Geometry: final body of the model. Coordinates: model frame, mm. A direction names the side the tool comes from. Give positions to 0.01 mm unless a question says otherwise; leave off trailing zeros. Order: outer loops, then holes, each group sorted by start corner. A loop starts at its lowest first (then second) coordinate and runs counter-clockwise, first axis right, second up. Notation, with made-up numbers: (27.5, 37.25) -> (55.5, 37.25) arc R28 cw to (55.5, 58.25) -> close; hole circle Ø11 at (81.25, -37.5). An arc over 180 degrees is marked (long way). One line per question, with ' | ' between items. Start each with the question number.
(1) Mould query, pull axis Y, two halves, no side actions, for faces 6 (the face through (18.71, 62, 25)), 7 (the face through (53, -14.773, 24)), 8 (the face through (53, 23.364, 17)), 9 (the face through (-11, 68.064, 17)). Classes: +Y half, -Y half, draft (parallel to the pull), parting line (faces both ways), or undercut.
(2) Section B-B (y = -19.5). Return loops of the section in (x, z).
(3) Section A-A (z = 5). Return loops of the section in (x, y), then the cut area to 3 significant figures.
(4) Ray query, L1, parallel to Y at x = -70, z = 18.5; L2, parallel to Y at x = -71, z = 3; L3, parallel to X at y = 50, z = 27. Return the intervals inside material, ascending.
(5) Set-up query: faces 1 (the face through (55, 33.196, 17)), 2 (the face through (-56.21, 50, 17)), 3 (the face through (-73, 23.228, 17)), 4 (the face through (-68.23, -26, 23)), 5 (the face through (-78.23, 26, 17)). Return all of +Z, -Z, +X, -X, +Y, -Y with unobstructed straight access to the full face (end or side cutting, diameter ignored); none if empty.
(6) Section C-C (x = -40.5). Return loops of the section in (y, z).
(7) First-contact query: pin 1 Ø7.5 at (y, z) = (18.5, 17) entering from +X; pin 2 Ø1 at (y, z) = (-20, 27) entering from -X; pin 3 Ø3.5 at (y, z) = (30, 16) entering from -X; pin 4 Ø8.5 at (y, z) = (53, 22.5) entering from -X. Flat tips, straight axial feed; report the tip coordinate or a pass-through.
```python
from build123d import *

# Parameters (mm, degrees)
SKETCH_1_W           = 136.18
SKETCH_1_H           = 105.19
EXTRUDE_1_DEPTH      = 34
SKETCH_3_W           = 39.24
SKETCH_3_H           = 34
CUT_EXTRUDE_1_DEPTH  = 28.96
SKETCH_4_W           = 17.22
SKETCH_4_H           = 34
EXTRUDE_2_DEPTH      = 17.22
SKETCH_5_W           = 19.62
SKETCH_5_H           = 34
EXTRUDE_3_DEPTH      = 17.22
SKETCH_6_W           = 34
SKETCH_6_H           = 4.24
CUT_EXTRUDE_2_DEPTH  = 5
SKETCH_7_W           = 34
SKETCH_7_H           = 7
CUT_EXTRUDE_4_DEPTH  = 10
SKETCH_9_W           = 19.62
SKETCH_9_H           = 13.59
EXTRUDE_4_DEPTH      = 11
SKETCH_10_W          = 17.22
SKETCH_10_H          = 13.58
EXTRUDE_5_DEPTH      = 11
SKETCH_11_W          = 34
SKETCH_11_H          = 5
CUT_EXTRUDE_7_DEPTH  = 5
SKETCH_13_W          = 33.75
SKETCH_13_H          = 7
CUT_EXTRUDE_9_DEPTH  = 10
SKETCH_15_W          = 10
SKETCH_15_H          = 7
CUT_EXTRUDE_10_DEPTH = 10
SKETCH_16_W          = 21.544160933
SKETCH_16_H          = 22.857254915
CUT_EXTRUDE_11_DEPTH = 10
SKETCH_18_W          = 19.981240116
SKETCH_18_H          = 22.352912948
CUT_EXTRUDE_12_DEPTH = 10


with BuildPart() as part:
    # 草图1 → 凸台-拉伸1 (new body)
    with BuildSketch(Plane.XY):
        with Locations((-10.139734918, 15.469024107)):
            Rectangle(SKETCH_1_W, SKETCH_1_H)
    extrude(amount=EXTRUDE_1_DEPTH)

    # 草图3 → 切除-拉伸1 (cut)
    with BuildSketch(Plane(origin=(0, 68.064024107, 0), x_dir=(1, 0, 0), z_dir=(0, 1, 0))):
        with Locations((-58.609734918, -17)):
            Rectangle(SKETCH_3_W, SKETCH_3_H)
        with Locations((38.330265082, -17)):
            Rectangle(SKETCH_3_W, SKETCH_3_H)
    extrude(amount=-CUT_EXTRUDE_1_DEPTH, mode=Mode.SUBTRACT)

    # 草图4 → 凸台-拉伸2 (add)
    with BuildSketch(Plane(origin=(0, 39.104024107, 0), x_dir=(1, 0, 0), z_dir=(0, 1, 0))):
        with Locations((-47.599734918, -17)):
            Rectangle(SKETCH_4_W, SKETCH_4_H)
    extrude(amount=EXTRUDE_2_DEPTH)

    # 草图5 → 凸台-拉伸3 (add)
    with BuildSketch(Plane(origin=(0, 39.104024107, 0), x_dir=(1, 0, 0), z_dir=(0, 1, 0))):
        with Locations((28.520265082, -17)):
            Rectangle(SKETCH_5_W, SKETCH_5_H)
    extrude(amount=EXTRUDE_3_DEPTH)

    # 草图6 → 切除-拉伸2 (cut)
    with BuildSketch(Plane.ZY.offset(78.229734918)):
        with Locations((17, 30.112750363)):
            Rectangle(SKETCH_6_W, SKETCH_6_H)
    extrude(amount=-CUT_EXTRUDE_2_DEPTH, mode=Mode.SUBTRACT)

    # 草图7 → 切除-拉伸4 (cut)
    with BuildSketch(Plane.ZY.offset(78.229734918)):
        with Locations((17, 19.728275547)):
            Rectangle(SKETCH_7_W, SKETCH_7_H)
    extrude(amount=-CUT_EXTRUDE_4_DEPTH, mode=Mode.SUBTRACT)

    # 草图9 → 凸台-拉伸4 (add)
    with BuildSketch(Plane(origin=(0, 56.324024107, 0), x_dir=(1, 0, 0), z_dir=(0, 1, 0))):
        with Locations((28.520265082, -6.795)):
            Rectangle(SKETCH_9_W, SKETCH_9_H)
    extrude(amount=EXTRUDE_4_DEPTH)

    # 草图10 → 凸台-拉伸5 (add)
    with BuildSketch(Plane(origin=(0, 56.324024107, 0), x_dir=(1, 0, 0), z_dir=(0, 1, 0))):
        with Locations((-47.599734918, -6.79)):
            Rectangle(SKETCH_10_W, SKETCH_10_H)
    extrude(amount=EXTRUDE_5_DEPTH)

    # 草图11 → 切除-拉伸7 (cut)
    with BuildSketch(Plane(origin=(57.950265082, 0, 0), x_dir=(0, 0, -1), z_dir=(1, 0, 0))):
        with Locations((-17, 30.695910163)):
            Rectangle(SKETCH_11_W, SKETCH_11_H)
    extrude(amount=-CUT_EXTRUDE_7_DEPTH, mode=Mode.SUBTRACT)

    # 草图13 → 切除-拉伸9 (cut)
    with BuildSketch(Plane(origin=(57.950265082, 0, 0), x_dir=(0, 0, -1), z_dir=(1, 0, 0))):
        with Locations((-16.874526915, 19.863616172)):
            Rectangle(SKETCH_13_W, SKETCH_13_H)
    extrude(amount=-CUT_EXTRUDE_9_DEPTH, mode=Mode.SUBTRACT)

    # 草图15 → 切除-拉伸10 (cut)
    with BuildSketch(Plane(origin=(0, 0, 33.749526915), x_dir=(-1, 0, 0), z_dir=(0, 0, -1))):
        with Locations((-52.950265082, 19.863616172)):
            Rectangle(SKETCH_15_W, SKETCH_15_H)
    extrude(amount=-CUT_EXTRUDE_10_DEPTH, mode=Mode.SUBTRACT)

    # 草图16 → 切除-拉伸11 (cut)
    with BuildSketch(Plane.ZY.offset(78.229734918)):
        with Locations((23.227919533, -25.697348436)):
            Rectangle(SKETCH_16_W, SKETCH_16_H)
    extrude(amount=-CUT_EXTRUDE_11_DEPTH, mode=Mode.SUBTRACT)

    # 草图18 → 切除-拉伸12 (cut)
    with BuildSketch(Plane(origin=(57.950265082, 0, 0), x_dir=(0, 0, -1), z_dir=(1, 0, 0))):
        with Locations((-24.009379942, -25.949519419)):
            Rectangle(SKETCH_18_W, SKETCH_18_H)
    extrude(amount=-CUT_EXTRUDE_12_DEPTH, mode=Mode.SUBTRACT)


solid = part.part
```
Response:
1) face 6: draft | face 7: -Y half | face 8: undercut | face 9: +Y half
2) outline: (-78.23, 0) -> (57.95, 0) -> (57.95, 14.02) -> (47.95, 14.02) -> (47.95, 34) -> (-68.23, 34) -> (-68.23, 12.46) -> (-78.23, 12.46) -> close
3) outline: (-78.23, -37.13) -> (57.95, -37.13) -> (57.95, 16.36) -> (47.95, 16.36) -> (47.95, 23.36) -> (57.95, 23.36) -> (57.95, 28.2) -> (52.95, 28.2) -> (52.95, 33.2) -> (57.95, 33.2) -> (57.95, 39.1) -> (38.33, 39.1) -> (38.33, 67.32) -> (18.71, 67.32) -> (18.71, 68.06) -> (-38.99, 68.06) -> (-38.99, 67.32) -> (-56.21, 67.32) -> (-56.21, 39.1) -> (-78.23, 39.1) -> (-78.23, 32.23) -> (-73.23, 32.23) -> (-73.23, 27.99) -> (-78.23, 27.99) -> (-78.23, 23.23) -> (-68.23, 23.23) -> (-68.23, 16.23) -> (-78.23, 16.23) -> close | area: 12,900 mm^2
4) L1: y = -14.27 to 16.23, 23.23 to 39.1 | L2: y = -37.13 to 16.23, 23.23 to 39.1 | L3: x = -56.21 to 38.33
5) face 1: +Z, -Z, +X | face 2: +Z, -Z, -X, +Y | face 3: +Z, -Z, -X | face 4: +Z, -X, -Y | face 5: +Z, -Z, -X, +Y, -Y
6) outline: (-37.13, 0) -> (67.32, 0) -> (67.32, 13.58) -> (56.32, 13.58) -> (56.32, 34) -> (-37.13, 34) -> close
7) pin 1: stops at x = 57.95 | pin 2: stops at x = -68.23 | pin 3: stops at x = -73.23 | pin 4: stops at x = -56.21
